Drawing for the job (mm, zero at the part's lowest x, y, z). A direction names the side the tool comes from. Give positions to 0.01 mm unless a question says otherwise; leave off trailing zeros. Write each loop counter-clockwise with the first axis right and the second up, starting at its lowest first coordinate (ties: lowest second). Pieces come first, ordered by that corner, then holes. Notation, with made-up numbers: M -36,3.5 L -8,3.5 A26 cw -8,36.5 Z; hole C 41.25,8 d7. An arc over 180 degrees is marked long. Use CSV: the item, a comma, the result in double quotes. Start each with the question number.
1. Drill centre lines: line 1 along Y through (x, z) = (8.5, 3); line 2 along Y through (x, z) = (3, 2); line 3 along Y through (x, z) = (3.5, 2). Where is each one in solid material? Low to high. Write a range as from..to.
2. Drop a flat-ended pin along its axis: pin 1 Ø2 at (y, z) = (2.5, 3) entering from -X. Give the stop position or say it passes through.
3. Band-saw the part on B-B, the plane z = 3. List the corners of the cut face in (x, y), then the cut area to 3 significant figures.
4. Band-saw the part on D-D, the plane x = 6.75. List the corners of the cut face in (y, z), then the cut area to 3 significant figures.
5. Band-saw the part on C-C, the plane x = 4.5. List the corners of the cut face in (y, z).
6. Mould opens along Z. For the marked faces 3, 4 and 5 say: pulls with the +Z half, pulls with the -Z half, needs draft (parallel to the pull), parting line crosses it, or undercut.
7. Band-saw the part on A-A, the plane y = 2.5. List the corners of the cut face in (x, z), then the cut area to 3 significant figures.
8. 3-axis set-ups, long thin cutter, end or side, ignore diameter. For the marked faces 1 and 2: which of +Z, -Z, +X, -X, +Y, -Y reach the whole face in a straight line?
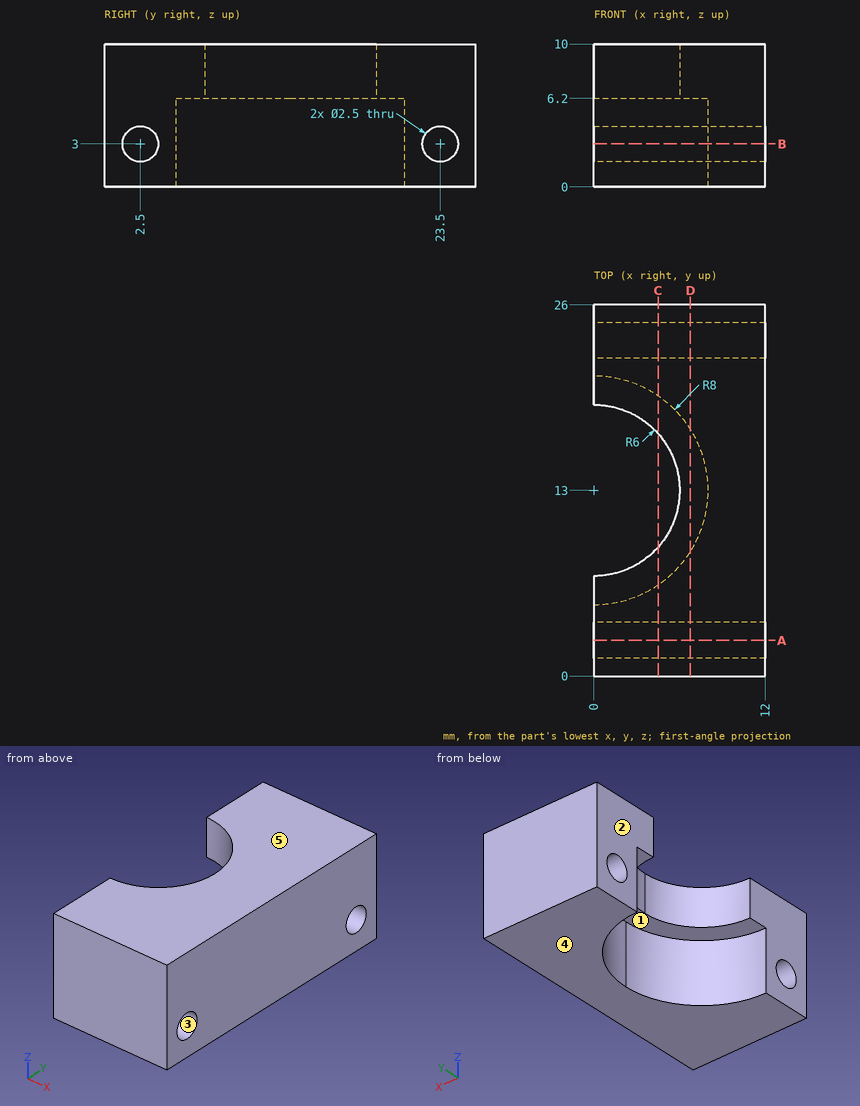
Output:
1,line 1,"y = 0..1.25, 3.75..22.25, 24.75..26"
1,line 2,"y = 0..1.75, 3.25..5.58, 20.42..22.75, 24.25..26"
1,line 3,"y = 0..1.75, 3.25..5.81, 20.19..22.75, 24.25..26"
2,pin 1,"passes through"
3,outline,"M 0,0 L 12,0 L 12,1.25 L 0,1.25 Z; M 0,3.75 L 12,3.75 L 12,22.25 L 0,22.25 L 0,21 A8 cw 0,5 Z; M 0,24.75 L 12,24.75 L 12,26 L 0,26 Z"
3,area,"151 mm²"
4,outline,"M 0,0 L 8.71,0 L 8.71,6.2 L 17.29,6.2 L 17.29,0 L 26,0 L 26,10 L 0,10 Z; hole C 2.5,3 d2.5; hole C 23.5,3 d2.5"
4,area,"197 mm²"
5,outline,"M 0,0 L 6.39,0 L 6.39,6.2 L 9.03,6.2 L 9.03,10 L 0,10 Z; M 16.97,6.2 L 19.61,6.2 L 19.61,0 L 26,0 L 26,10 L 16.97,10 Z; hole C 2.5,3 d2.5; hole C 23.5,3 d2.5"
6,face 3,"undercut"
6,face 4,"pulls with the -Z half"
6,face 5,"pulls with the +Z half"
7,outline,"M 0,0 L 12,0 L 12,1.75 L 0,1.75 Z; M 0,4.25 L 12,4.25 L 12,10 L 0,10 Z"
7,area,"90.0 mm²"
8,face 1,"-Z, -X"
8,face 2,"+Z, -Z, -X, +Y, -Y"
